from build123d import *

# Parameters (mm, degrees)
SKETCH2_R           = 15
BOSS_EXTRUDE1_DEPTH = 10
BOSS_EXTRUDE2_DEPTH = 6
SKETCH4_R           = 2.5
CUT_EXTRUDE1_DEPTH  = 8
SKETCH6_W           = 0.825946649
SKETCH6_H           = 5.007301559
BOSS_EXTRUDE3_DEPTH = 15


with BuildPart() as part:
    # Sketch2 → Boss-Extrude1 (new body)
    with BuildSketch(Plane(origin=(0, 0, 0), x_dir=(0, 0, -1), z_dir=(1, 0, 0))):
        Circle(SKETCH2_R)
    extrude(amount=BOSS_EXTRUDE1_DEPTH)

    # Sketch3 → Boss-Extrude2 (add)
    with BuildSketch(Plane(origin=(10, 0, 0), x_dir=(0, 0, -1), z_dir=(1, 0, 0))):
        with BuildLine():
            Line((-10, 3.5), (10, 3.5))
            ThreePointArc((10, 3.5), (13.5, 0), (10, -3.5))
            Line((10, -3.5), (-10, -3.5))
            ThreePointArc((-10, -3.5), (-13.5, 0), (-10, 3.5))
        make_face()
    extrude(amount=BOSS_EXTRUDE2_DEPTH)

    # Sketch4 → Cut-Extrude1 (cut)
    with BuildSketch(Plane.ZY):
        Circle(SKETCH4_R)
    extrude(amount=-CUT_EXTRUDE1_DEPTH, mode=Mode.SUBTRACT)

    # Sketch6 → Boss-Extrude3 (add)
    with BuildSketch(Plane.ZY.offset(-8)):
        with Locations((-0.025810832, -0.051621665)):
            Rectangle(SKETCH6_W, SKETCH6_H)
    extrude(amount=BOSS_EXTRUDE3_DEPTH)


solid = part.part
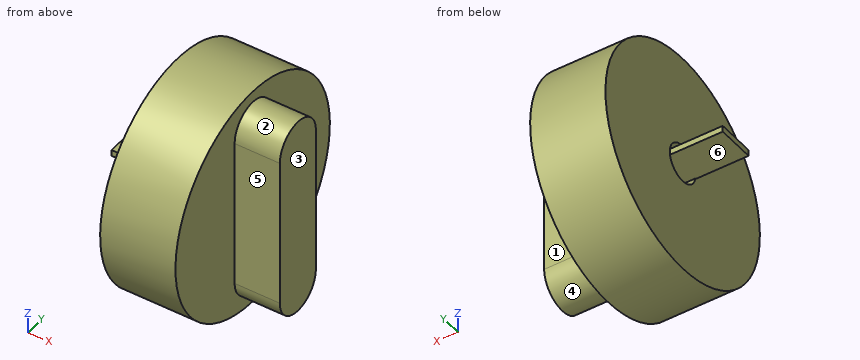
Input: part model. Units: mm. Frame: model coordinates. Face numbers are marked on the shaded views. A direction names the side the tool comes from. Coordinates: 2 decimals unless noted, no trailing zeros. Order: outer loops, then holes, each group sorted by start corner. A loop starts at its lowest first (then second) coordinate and runs counter-clockwise, first axis right, second up. Notation, with made-up numbers: M 60,-35 L 88,-35 A25 ccw 88,2 Z; hole C 67,-34.75 d11. An arc over 180 degrees is marked long. Write item = value, one per line. Start each with the question number.
(1) Section B-B on z = 0. Output: boundary loops of the cut face in (x, y).
(2) Pull-direction query (Y, two-part tool) for the marked faces 4, 5 and 6; classes: released by +Y, released by -Y, zero draft, split by the parting line, or undercut.
(3) Section D-D on x = 7. Output: boundary loops of the cut face in (y, z), and give its area (3 significant figures).
(4) First-contact query: P1, Ø1.5, axis at x = 0.5, z = 6.5, coming from the +Y side; P2, Ø3, axis at x = 14, z = 1.5, coming from the -Y side; P3, Ø4, axis at x = -3.5, z = 8, coming from the -Y side; P4, Ø8, axis at y = 8.5, z = -11.5, coming from the -X side. Flat tips, straight axial feed; report the tip coordinate or a pass-through.
(5) Reachability of the marked faces 1, 2 and 3 from +Z, -Z, +X, -X, +Y, -Y: full face, straight path, thin tool, end or side. Return the list, or none.
(6) Section A-A on y = 0. Output: boundary loops of the cut face in (x, z), and give its area (3 significant figures).
(7) Line query: line 1 along X through (y, z) = (-12.25, 4.5); line 2 along X through (y, z) = (2, -2); line 3 along Z through (x, y) = (8.75, 4.25). Output: solid intervals per line, ascending. Write a range as [from, to].
(8) Section C-C on x = -4. Output: boundary loops of the cut face in (y, z).
Result set:
q1.outline = M -7,-2.56 L 0,-2.56 L 0,-15 L 10,-15 L 10,-3.5 L 16,-3.5 L 16,3.5 L 10,3.5 L 10,15 L 0,15 L 0,2.5 L 8,2.5 L 8,2.45 L -7,2.45 Z
q2.face_4 = split by the parting line
q2.face_5 = released by -Y
q2.face_6 = undercut
q3.outline = C 0,0 d30; hole M -2.47,0.39 L 2.45,0.39 L 2.45,-0.44 L -2.46,-0.44 A2.5 ccw long Z
q3.area = 691 mm²
q4.P1 = 13.85
q4.P2 = -3.5
q4.P3 = through
q4.P4 = 0
q5.face_1 = +Z, -Z, +X, +Y
q5.face_2 = +Z, +X
q5.face_3 = +Z, -Z, +X, +Y, -Y
q6.outline = M -7,-0.44 L 8,-0.44 L 8,-2.5 L 0,-2.5 L 0,-15 L 10,-15 L 10,-13.5 L 16,-13.5 L 16,13.5 L 10,13.5 L 10,15 L 0,15 L 0,2.5 L 8,2.5 L 8,0.39 L -7,0.39 Z
q6.area = 434 mm²
q7.line_1 = [0, 10]
q7.line_2 = [0, 16]
q7.line_3 = [-14.39, 14.39]
q8.outline = M -2.56,-0.44 L 2.45,-0.44 L 2.45,0.39 L -2.56,0.39 Z
